Here's how the part is built. I have some questions about the finished solid (model axes, mm). Give positions to 0.01 mm unless a question says otherwise; leave off trailing zeros. Write each loop counter-clockwise with the first axis right and the second up, starting at its lowest first coordinate (ties: lowest second). Pieces come first, ordered by that corner, then holes. Notation, with made-up numbers: M 26.25,-8 L 75.25,-8 A29 ccw 75.25,13 Z; hole C 36.5,15 d1. An arc over 180 degrees is marked long. Answer as CSV lines item,"result". Start each with the question number.
Q1. Suppose I cut it at B-B (y = -3.5). Write out the boundary of the cut face in (x, z).
Q2. For pin 1 (0.8 mm diameter, centred on x = 8.5, z = -1, fed in from -Y); pin 2 (12 mm diameter, centred on x = -31, y = -31.5, fed in from -Z); pin 3 (1.6 mm diameter, centred on y = -2, z = -1, fed in from -X), each with a flat end and sliding along its axis, tell me the tip position at first contact or that it passes through.
Q3. If I drill on line 1 along X through (y, z) = (4, 0.9); line 2 along Z through (x, y) = (-11, 15); line 3 along Y through (x, z) = (18.5, 2.1), over which ranges is the centre line in solid material (lowest first)?
Q4. Suppose I cut it at A-A (x = -0.5). Write out the boundary of the cut face in (y, z), then the cut area to 3 significant figures.
Q5. Suppose I cut it at D-D (y = -29.5). Write out the boundary of the cut face in (x, z), then the cut area to 3 significant figures.
Q6. Suppose I cut it at C-C (x = -31). Write out the boundary of the cut face in (y, z).
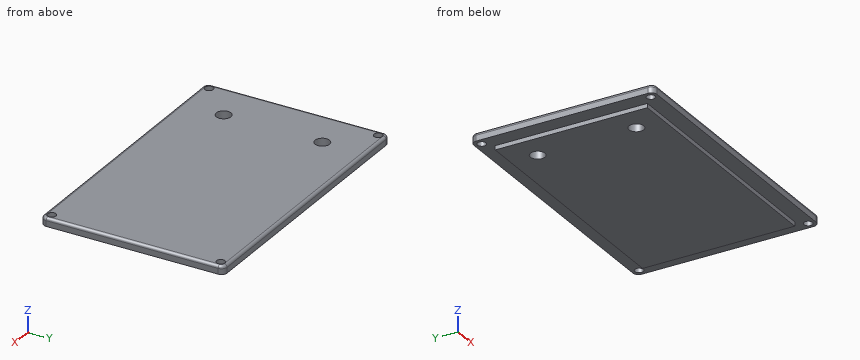
```python
from build123d import *

# Parameters (mm, degrees)
F0_W         = 100
F0_H         = 65
F0_R         = 1.5
F0_R_2       = 2.6
F1_DEPTH     = 3
F2_R         = 0.99999
F3_T1_DEPTH  = 8
F3_T4_ANGLE  = 90
F3_T6_ANGLE  = 90
F3_T8_ANGLE  = 90
F3_T10_ANGLE = 90
F4_W         = 89
F4_H         = 54
F4_R         = 2.6
F5_DEPTH     = 1.5


# Not quite as in the source:
# - a fillet or chamfer that OpenCascade refuses, or shapes differently, is made with other operations: its cross-section is extruded or revolved along the edge and cut away or added
# - a fillet or chamfer is up to 0.001 mm smaller than in the source, because OpenCascade refuses the exact size


with BuildPart() as f1:
    # F0 (on Top) → F1 (new body)
    with BuildSketch(Plane.XY):
        with Locations((4.8531983048, -13.4167700263)):
            Rectangle(F0_W, F0_H)
        with Locations((-42.6468016952, -43.4167700263)):
            Circle(F0_R, mode=Mode.SUBTRACT)
        with Locations((-30.1468016952, -30.9167700263)):
            Circle(F0_R_2, mode=Mode.SUBTRACT)
        with Locations((52.3531983048, -43.4167700263)):
            Circle(F0_R, mode=Mode.SUBTRACT)
        with Locations((-30.1468016952, 4.0832299737)):
            Circle(F0_R_2, mode=Mode.SUBTRACT)
        with Locations((-42.6468016952, 16.5832299737)):
            Circle(F0_R, mode=Mode.SUBTRACT)
        with Locations((52.3531983048, 16.5832299737)):
            Circle(F0_R, mode=Mode.SUBTRACT)
    extrude(amount=F1_DEPTH)

    # F2 (radius 1 in the source; OpenCascade refuses exactly that, so slightly less here)
    f2_edges = [f1.edges().sort_by_distance(p)[0] for p in [
        (-45.146802, -13.41677, 3),
        (4.853198, 19.08323, 3),
        (54.853198, -13.41677, 3),
        (4.853198, -45.91677, 3),
    ]]
    fillet(f2_edges, radius=F2_R)

    # F3: fillet of radius 2 on 4 edges, made by hand

    # F3_s2 → F3_t1 (cut)
    with BuildSketch(Plane.XY.offset(-5)):
        with BuildLine():
            ThreePointArc((-43.1468016952, -45.9167700263), (-44.5610152576, -45.3309835887), (-45.1468016952, -43.9167700263))
            Line((-45.1468016952, -43.9167700263), (-45.1468016952, -45.9167700263))
            Line((-45.1468016952, -45.9167700263), (-43.1468016952, -45.9167700263))
        make_face()
        with BuildLine():
            ThreePointArc((-43.1468016952, 19.0832299737), (-44.5610152576, 18.4974435361), (-45.1468016952, 17.0832299737))
            Line((-45.1468016952, 17.0832299737), (-45.1468016952, 19.0832299737))
            Line((-45.1468016952, 19.0832299737), (-43.1468016952, 19.0832299737))
        make_face()
        with BuildLine():
            ThreePointArc((54.8531983048, 17.0832299737), (54.2674118671, 18.4974435361), (52.8531983048, 19.0832299737))
            Line((52.8531983048, 19.0832299737), (54.8531983048, 19.0832299737))
            Line((54.8531983048, 19.0832299737), (54.8531983048, 17.0832299737))
        make_face()
        with BuildLine():
            ThreePointArc((54.8531983048, -43.9167700263), (54.2674118671, -45.3309835887), (52.8531983048, -45.9167700263))
            Line((52.8531983048, -45.9167700263), (54.8531983048, -45.9167700263))
            Line((54.8531983048, -45.9167700263), (54.8531983048, -43.9167700263))
        make_face()
    extrude(amount=F3_T1_DEPTH, mode=Mode.SUBTRACT)

    # F3_s3 → F3_t4 (revolve, cut)
    with BuildSketch(Plane.YZ.offset(52.8531983048)):
        with BuildLine():
            ThreePointArc((-44.9167800263, 3), (-45.6238797364, 2.7071097101), (-45.9167700263, 2.00001))
            Line((-45.9167700263, 2.00001), (-45.9167700263, 3))
            Line((-45.9167700263, 3), (-44.9167800263, 3))
        make_face()
    revolve(axis=Axis((52.8531983048, -43.9167700263, 3), (0, 0, 1)), revolution_arc=F3_T4_ANGLE, mode=Mode.SUBTRACT)

    # F3_s5 → F3_t6 (revolve, cut)
    with BuildSketch(Plane.XZ.offset(-17.0832299737)):
        with BuildLine():
            ThreePointArc((53.8532083048, 3), (54.5603080149, 2.7071097101), (54.8531983048, 2.00001))
            Line((54.8531983048, 2.00001), (54.8531983048, 3))
            Line((54.8531983048, 3), (53.8532083048, 3))
        make_face()
    revolve(axis=Axis((52.8531983048, 17.0832299737, 3), (0, 0, 1)), revolution_arc=F3_T6_ANGLE, mode=Mode.SUBTRACT)

    # F3_s7 → F3_t8 (revolve, cut)
    with BuildSketch(Plane.YZ.offset(-43.1468016952)):
        with BuildLine():
            ThreePointArc((18.0832399737, 3), (18.7903396838, 2.7071097101), (19.0832299737, 2.00001))
            Line((19.0832299737, 2.00001), (19.0832299737, 3))
            Line((19.0832299737, 3), (18.0832399737, 3))
        make_face()
    revolve(axis=Axis((-43.1468016952, 17.0832299737, 3), (0, 0, 1)), revolution_arc=F3_T8_ANGLE, mode=Mode.SUBTRACT)

    # F3_s9 → F3_t10 (revolve, cut)
    with BuildSketch(Plane.XZ.offset(43.9167700263)):
        with BuildLine():
            ThreePointArc((-44.1468116952, 3), (-44.8539114053, 2.7071097101), (-45.1468016952, 2.00001))
            Line((-45.1468016952, 2.00001), (-45.1468016952, 3))
            Line((-45.1468016952, 3), (-44.1468116952, 3))
        make_face()
    revolve(axis=Axis((-43.1468016952, -43.9167700263, 3), (0, 0, 1)), revolution_arc=F3_T10_ANGLE, mode=Mode.SUBTRACT)

    # F4 (on face) → F5 (join)
    with BuildSketch(Plane(origin=(0, 0, 0), x_dir=(1, 0, 0), z_dir=(0, 0, -1))):
        with Locations((4.8531983048, 13.4167700263)):
            Rectangle(F4_W, F4_H)
        with Locations((-30.1468016952, -4.0832299737)):
            Circle(F4_R, mode=Mode.SUBTRACT)
        with Locations((-30.1468016952, 30.9167700263)):
            Circle(F4_R, mode=Mode.SUBTRACT)
    extrude(amount=F5_DEPTH)


solid = f1.part
```
Resolved:
1,outline,"M -45.15,0 L -39.65,0 L -39.65,-1.5 L 49.35,-1.5 L 49.35,0 L 54.85,0 L 54.85,2 A1 ccw 53.85,3 L -44.15,3 A1 ccw -45.15,2 Z"
2,pin 1,"y = -40.42"
2,pin 2,"z = -1.5"
2,pin 3,"x = -39.65"
3,line 1,"-45.15 to -32.75, -27.55 to 54.85"
3,line 2,"0 to 3"
3,line 3,"-45.91 to 19.08"
4,outline,"M -45.92,0 L -40.42,0 L -40.42,-1.5 L 13.58,-1.5 L 13.58,0 L 19.08,0 L 19.08,2 A1 ccw 18.08,3 L -44.92,3 A1 ccw -45.92,2 Z"
4,area,"276 mm^2"
5,outline,"M -45.15,0 L -39.65,0 L -39.65,-1.5 L -32.33,-1.5 L -32.33,3 L -44.15,3 A1 ccw -45.15,2 Z; M -27.97,-1.5 L 49.35,-1.5 L 49.35,0 L 54.85,0 L 54.85,2 A1 ccw 53.85,3 L -27.97,3 Z"
5,area,"413 mm^2"
6,outline,"M -45.92,0 L -40.42,0 L -40.42,-1.5 L -33.37,-1.5 L -33.37,3 L -44.92,3 A1 ccw -45.92,2 Z; M -28.46,-1.5 L 1.63,-1.5 L 1.63,3 L -28.46,3 Z; M 6.54,-1.5 L 13.58,-1.5 L 13.58,0 L 19.08,0 L 19.08,2 A1 ccw 18.08,3 L 6.54,3 Z"
